from build123d import *

# Parameters (mm, degrees)
SKICA1_R                      = 250
P_IDAT_VYSUNUT_M1_DEPTH       = 50
SKICA2_R                      = 175
ODEBRAT_VYSUNUT_M1_DEPTH      = 60
ZAOBLIT1_R                    = 10
SKICA4_R                      = 7.5
ODEBRAT_VYSUNUT_M2_DEPTH      = 51
SKICA6_R                      = 7.5
ODEBRAT_VYSUNUT_M3_DEPTH      = 251
ODEBRAT_VYSUNUT_M3_DEPTH_BACK = 251


with BuildPart() as part:
    # Skica1 → Přidat vysunutím1 (new body)
    with BuildSketch(Plane(origin=(0, 0, 0), x_dir=(1, 0, 0), z_dir=(0, 1, 0))):
        with Locations(Location((0, 0, 0), (0, 0, 270))):  # turned: the seam where the file's is
            Circle(SKICA1_R)
    extrude(amount=-P_IDAT_VYSUNUT_M1_DEPTH)

    # Skica2 → Odebrat vysunutím1 (cut)
    with BuildSketch(Plane(origin=(0, 0, 0), x_dir=(1, 0, 0), z_dir=(0, 1, 0))):
        with Locations(Location((0, 0, 0), (0, 0, 270))):  # turned: the seam where the file's is
            Circle(SKICA2_R)
    extrude(amount=-ODEBRAT_VYSUNUT_M1_DEPTH, mode=Mode.SUBTRACT)

    # Zaoblit1
    zaoblit1_edges = [part.edges().sort_by_distance(p)[0] for p in [
        (0, 0, -250),
    ]]
    fillet(zaoblit1_edges, radius=ZAOBLIT1_R)

    # Skica4 → Odebrat vysunutím2 (cut, through all)
    with BuildSketch(Plane(origin=(0, 0, 0), x_dir=(1, 0, 0), z_dir=(0, 1, 0))):
        with Locations(Location((-25, -228.637267303, 0), (0, 0, 270))):  # turned: the seam where the file's is
            Circle(SKICA4_R)
        with Locations(Location((25, -228.637267303, 0), (0, 0, 90))):  # turned: the seam where the file's is
            Circle(SKICA4_R)
        with Locations(Location((-135.969268746, -185.505681737, 0), (0, 0, 270))):  # turned: the seam where the file's is
            Circle(SKICA4_R)
        with Locations(Location((-92.667998557, -210.505681737, 0), (0, 0, 90))):  # turned: the seam where the file's is
            Circle(SKICA4_R)
        with Locations(Location((-210.505681737, -92.667998557, 0), (0, 0, 270))):  # turned: the seam where the file's is
            Circle(SKICA4_R)
        with Locations(Location((-185.505681737, -135.969268746, 0), (0, 0, 90))):  # turned: the seam where the file's is
            Circle(SKICA4_R)
        with Locations(Location((-228.637267303, 25, 0), (0, 0, 270))):  # turned: the seam where the file's is
            Circle(SKICA4_R)
        with Locations(Location((-228.637267303, -25, 0), (0, 0, 90))):  # turned: the seam where the file's is
            Circle(SKICA4_R)
        with Locations(Location((-185.505681737, 135.969268746, 0), (0, 0, 270))):  # turned: the seam where the file's is
            Circle(SKICA4_R)
        with Locations(Location((-210.505681737, 92.667998557, 0), (0, 0, 90))):  # turned: the seam where the file's is
            Circle(SKICA4_R)
        with Locations(Location((-92.667998557, 210.505681737, 0), (0, 0, 270))):  # turned: the seam where the file's is
            Circle(SKICA4_R)
        with Locations(Location((-135.969268746, 185.505681737, 0), (0, 0, 90))):  # turned: the seam where the file's is
            Circle(SKICA4_R)
        with Locations(Location((25, 228.637267303, 0), (0, 0, 270))):  # turned: the seam where the file's is
            Circle(SKICA4_R)
        with Locations(Location((-25, 228.637267303, 0), (0, 0, 90))):  # turned: the seam where the file's is
            Circle(SKICA4_R)
        with Locations(Location((135.969268746, 185.505681737, 0), (0, 0, 270))):  # turned: the seam where the file's is
            Circle(SKICA4_R)
        with Locations(Location((92.667998557, 210.505681737, 0), (0, 0, 90))):  # turned: the seam where the file's is
            Circle(SKICA4_R)
        with Locations(Location((210.505681737, 92.667998557, 0), (0, 0, 270))):  # turned: the seam where the file's is
            Circle(SKICA4_R)
        with Locations(Location((185.505681737, 135.969268746, 0), (0, 0, 90))):  # turned: the seam where the file's is
            Circle(SKICA4_R)
        with Locations(Location((228.637267303, -25, 0), (0, 0, 270))):  # turned: the seam where the file's is
            Circle(SKICA4_R)
        with Locations(Location((228.637267303, 25, 0), (0, 0, 90))):  # turned: the seam where the file's is
            Circle(SKICA4_R)
        with Locations(Location((185.505681737, -135.969268746, 0), (0, 0, 270))):  # turned: the seam where the file's is
            Circle(SKICA4_R)
        with Locations(Location((210.505681737, -92.667998557, 0), (0, 0, 90))):  # turned: the seam where the file's is
            Circle(SKICA4_R)
        with Locations(Location((92.667998557, -210.505681737, 0), (0, 0, 270))):  # turned: the seam where the file's is
            Circle(SKICA4_R)
        with Locations(Location((135.969268746, -185.505681737, 0), (0, 0, 90))):  # turned: the seam where the file's is
            Circle(SKICA4_R)
    extrude(amount=-ODEBRAT_VYSUNUT_M2_DEPTH, mode=Mode.SUBTRACT)

    # Skica6 → Odebrat vysunutím3 (cut, two sides)
    with BuildSketch(Plane.XY) as odebrat_vysunut_m3_sk:
        with Locations((0, -20)):
            Circle(SKICA6_R)
    extrude(amount=ODEBRAT_VYSUNUT_M3_DEPTH, mode=Mode.SUBTRACT)
    extrude(odebrat_vysunut_m3_sk.sketch, amount=-ODEBRAT_VYSUNUT_M3_DEPTH_BACK, mode=Mode.SUBTRACT)


solid = part.part
Can you work these out from the model? Positions are in its coordinate system, mm. Round coordinates to 2 decimals unless told otherwise and drop trailing zeros. Write each loop counter-clockwise with the first axis right and the second up, starting at its lowest first coordinate (ties: lowest second). Pieces come first, ordered by that corner, then holes. Notation, with made-up numbers: (15, 35) - (47, 35) arc R29 cw to (47, 69) - close; hole circle Ø5 at (43.25, 10.25). An arc over 180 degrees is marked (long way). Write each question's results on one line, items separated by ' | '. Start each with the question number.
1) For pin 1 Ø17 at (x, z) = (-25, 228.64) entering from +Y; pin 2 Ø4 at (y, z) = (-29.5, -20.5) entering from +X; pin 3 Ø2 at (y, z) = (-21.5, 141) entering from -X; pin 4 Ø1.5 at (x, y) = (156, -6.5) entering from -Z, each with a flat end and sliding along its axis, tell me the tip position at first contact or that it passes through.
2) Suppose I cut it at B-B (x = 0). List the corners of the cut face in (y, z) for me, and give its area (3 significant figures).
3) We'd pull the mould along Z, two halves only. Please class faces 1 (the cylindrical face through (-0.976, -12.564, 211.893)), 2 (the cylindrical face through (140.53, -24.65, 191.46)), 3 (the cylindrical face through (10.99, -29.72, -249.76)): released by +Z, released by -Z, zero draft, split by the parting line, or undercut.
4) Suppose I cut it at C-C (y = -20). Give the number of separate pieces and of enclosed holes in the cut face, and give its area (3 significant figures).
5) Please list where these lines run through material, in increasing order: line 1 (X direction, y = -36.5, z = -25); line 2 (X direction, y = -33.5, z = 2.5); line 3 (X direction, y = -24.5, z = -30).
6) Suppose I cut it at A-A (z = 0). List the corners of the cut face in (x, y) for me.
Here are the results:
1) pin 1: stops at y = 0 | pin 2: stops at x = 249.31 | pin 3: stops at x = -207.12 | pin 4: stops at z = -195.23
2) outline: (-50, -250) - (-27.5, -250) - (-27.5, -175) - (-50, -175) - close; (-50, 175) - (-27.5, 175) - (-27.5, 250) - (-50, 250) - close; (-12.5, -250) - (-10, -250) arc R10 ccw to (0, -240) - (0, -175) - (-12.5, -175) - close; (-12.5, 175) - (0, 175) - (0, 240) arc R10 ccw to (-10, 250) - (-12.5, 250) - close | area: 5,210 mm2
3) face 1: zero draft | face 2: undercut | face 3: split by the parting line
4) separate pieces: 2 | enclosed holes: 24 | area: 93,600 mm2
5) line 1: x = -248.75 to -236.14, -221.14 to -173.21, 173.21 to 221.14, 236.14 to 248.75 | line 2: x = -249.99 to -174.98, 174.98 to 249.99 | line 3: x = -248.19 to -234.23, -223.05 to -172.41, 172.41 to 223.05, 234.23 to 248.19
6) outline: (-250, -50) - (-175, -50) - (-175, 0) - (-240, 0) arc R10 ccw to (-250, -10) - close; (175, -50) - (250, -50) - (250, -10) arc R10 ccw to (240, 0) - (175, 0) - close
